from build123d import *

# Parameters (mm, degrees)
SKETCH_1_R          = 2.65
SKETCH_1_R_2        = 1.5
EXTRUDE_1_DEPTH     = 52.7
SKETCH_4_R          = 3.1
CUT_EXTRUDE_3_DEPTH = 56.399571298


with BuildPart() as part:
    # 草图1 → 凸台-拉伸1 (new, symmetric)
    with BuildSketch(Plane.XY):
        with BuildLine():
            Line((3.142893219, 3.85), (-3.142893219, 3.85))
            Line((-3.142893219, 3.85), (-5.5, 6.207106781))
            Line((-5.5, 6.207106781), (-5.5, 8.3))
            Line((-5.5, 8.3), (-3.1, 8.3))
            Line((-3.1, 8.3), (-3.1, 9.5))
            Line((-3.1, 9.5), (-3.6, 9.5))
            Line((-3.6, 9.5), (-3.6, 9.7))
            ThreePointArc((-3.6, 9.7), (-3.687867966, 9.912132034), (-3.9, 10))
            Line((-3.9, 10), (-8.5, 10))
            ThreePointArc((-8.5, 10), (-9.560660172, 9.560660172), (-10, 8.5))
            Line((-10, 8.5), (-10, 3.9))
            ThreePointArc((-10, 3.9), (-9.912132034, 3.687867966), (-9.7, 3.6))
            Line((-9.7, 3.6), (-9.5, 3.6))
            Line((-9.5, 3.6), (-9.5, 3.1))
            Line((-9.5, 3.1), (-8.3, 3.1))
            Line((-8.3, 3.1), (-8.3, 5.5))
            Line((-8.3, 5.5), (-6.207106781, 5.5))
            Line((-6.207106781, 5.5), (-3.85, 3.142893219))
            Line((-3.85, 3.142893219), (-3.85, -3.142893219))
            Line((-3.85, -3.142893219), (-6.207106781, -5.5))
            Line((-6.207106781, -5.5), (-8.3, -5.5))
            Line((-8.3, -5.5), (-8.3, -3.1))
            Line((-8.3, -3.1), (-9.5, -3.1))
            Line((-9.5, -3.1), (-9.5, -3.6))
            Line((-9.5, -3.6), (-9.7, -3.6))
            ThreePointArc((-9.7, -3.6), (-9.912132034, -3.687867966), (-10, -3.9))
            Line((-10, -3.9), (-10, -8.5))
            ThreePointArc((-10, -8.5), (-9.560660172, -9.560660172), (-8.5, -10))
            Line((-8.5, -10), (-3.9, -10))
            ThreePointArc((-3.9, -10), (-3.687867966, -9.912132034), (-3.6, -9.7))
            Line((-3.6, -9.7), (-3.6, -9.5))
            Line((-3.6, -9.5), (-3.1, -9.5))
            Line((-3.1, -9.5), (-3.1, -8.3))
            Line((-3.1, -8.3), (-5.5, -8.3))
            Line((-5.5, -8.3), (-5.5, -6.207106781))
            Line((-5.5, -6.207106781), (-3.142893219, -3.85))
            Line((-3.142893219, -3.85), (3.142893219, -3.85))
            Line((3.142893219, -3.85), (5.5, -6.207106781))
            Line((5.5, -6.207106781), (5.5, -8.3))
            Line((5.5, -8.3), (3.1, -8.3))
            Line((3.1, -8.3), (3.1, -9.5))
            Line((3.1, -9.5), (3.6, -9.5))
            Line((3.6, -9.5), (3.6, -9.7))
            ThreePointArc((3.6, -9.7), (3.687867966, -9.912132034), (3.9, -10))
            Line((3.9, -10), (8.5, -10))
            ThreePointArc((8.5, -10), (9.560660172, -9.560660172), (10, -8.5))
            Line((10, -8.5), (10, -3.9))
            ThreePointArc((10, -3.9), (9.912132034, -3.687867966), (9.7, -3.6))
            Line((9.7, -3.6), (9.5, -3.6))
            Line((9.5, -3.6), (9.5, -3.1))
            Line((9.5, -3.1), (8.3, -3.1))
            Line((8.3, -3.1), (8.3, -5.5))
            Line((8.3, -5.5), (6.207106781, -5.5))
            Line((6.207106781, -5.5), (3.85, -3.142893219))
            Line((3.85, -3.142893219), (3.85, 3.142893219))
            Line((3.85, 3.142893219), (6.207106781, 5.5))
            Line((6.207106781, 5.5), (8.3, 5.5))
            Line((8.3, 5.5), (8.3, 3.1))
            Line((8.3, 3.1), (9.5, 3.1))
            Line((9.5, 3.1), (9.5, 3.6))
            Line((9.5, 3.6), (9.7, 3.6))
            ThreePointArc((9.7, 3.6), (9.912132034, 3.687867966), (10, 3.9))
            Line((10, 3.9), (10, 8.5))
            ThreePointArc((10, 8.5), (9.560660172, 9.560660172), (8.5, 10))
            Line((8.5, 10), (3.9, 10))
            ThreePointArc((3.9, 10), (3.687867966, 9.912132034), (3.6, 9.7))
            Line((3.6, 9.7), (3.6, 9.5))
            Line((3.6, 9.5), (3.1, 9.5))
            Line((3.1, 9.5), (3.1, 8.3))
            Line((3.1, 8.3), (5.5, 8.3))
            Line((5.5, 8.3), (5.5, 6.207106781))
            Line((5.5, 6.207106781), (3.142893219, 3.85))
        make_face()
        with Locations(Location((0, 0, 0), (0, 0, 180))):
            Circle(SKETCH_1_R, mode=Mode.SUBTRACT)
        with Locations(Location((-7.75, 7.75, 0), (0, 0, 180))):
            Circle(SKETCH_1_R_2, mode=Mode.SUBTRACT)
        with Locations(Location((7.75, 7.75, 0), (0, 0, 180))):
            Circle(SKETCH_1_R_2, mode=Mode.SUBTRACT)
        with Locations(Location((7.75, -7.75, 0), (0, 0, 180))):
            Circle(SKETCH_1_R_2, mode=Mode.SUBTRACT)
        with Locations(Location((-7.75, -7.75, 0), (0, 0, 180))):
            Circle(SKETCH_1_R_2, mode=Mode.SUBTRACT)
    extrude(amount=EXTRUDE_1_DEPTH, both=True)

    # 草图4 → 切除-拉伸3 (cut, through all)
    with BuildSketch(Plane(origin=(3.85, 0, 0), x_dir=(0, 0, -1), z_dir=(1, 0, 0))):
        with Locations((-38.1, 0)):
            Circle(SKETCH_4_R)
        with Locations((38.1, 0)):
            Circle(SKETCH_4_R)
    extrude(amount=-CUT_EXTRUDE_3_DEPTH, mode=Mode.SUBTRACT)


solid = part.part
Part model, mm, in its own coordinate system. A direction names the side the tool comes from. Give positions to 0.01 mm unless a question says otherwise; leave off trailing zeros. Loops run counter-clockwise (first coordinate to the right, second up) from the corner with the lowest first, then second, coordinate; pieces in that order, holes last.
(1) Band-saw the part on B-B (x = 0). Write the cut outline in (y, z), and give its area (3 significant figures).
Return value:
outline: (-3.85, -52.7) - (-2.65, -52.7) - (-2.65, -39.71) arc R3.1 cw to (-2.65, -36.49) - (-2.65, 36.49) arc R3.1 cw to (-2.65, 39.71) - (-2.65, 52.7) - (-3.85, 52.7) - close; (2.65, -52.7) - (3.85, -52.7) - (3.85, 52.7) - (2.65, 52.7) - (2.65, 39.71) arc R3.1 cw to (2.65, 36.49) - (2.65, -36.49) arc R3.1 cw to (2.65, -39.71) - close
area: 249 mm2
(2) Pin check, flat tips, straight feed: pin 1 (8 mm diameter, centred on y = 0, z = 25, fed in from +X); pin 2 (0.6 mm diameter, centred on x = 3.5, z = 3.5, fed in from -Y). Stop position of each tip, or through.
Return value:
pin 1: stops at x = 10
pin 2: stops at y = -9.98
(3) Drill centre lines: line 1 along Y through (x, z) = (7.75, -22); line 2 along X through (y, z) = (-9, 22). Where is each one in solid material? Low to high.
Return value:
line 1: y = -10 to -9.25, -6.25 to -5.5, 5.5 to 6.25, 9.25 to 10
line 2: x = -9.91 to -8.58, -6.92 to -3.1, 3.1 to 6.92, 8.58 to 9.91
(4) Band-saw the part on C-C (z = 38.1). Count the separate pieces of the cut face and the enclosed holes in it, and give its area (3 significant figures).
Return value:
separate pieces: 2
enclosed holes: 4
area: 104 mm2
(5) Pull direction Y, two halves, no side cores. Call faces 1 (the flat face through (-10, 6, 1)), 2 (the flat face through (-5.012, -4.305, 0.738)), 3 (the flat face through (-6, 10, 1)): pulls with the +Y half, pulls with the -Y half, needs draft (parallel to the pull), parting line crosses it, or undercut.
Return value:
face 1: needs draft
face 2: undercut
face 3: pulls with the +Y half
(6) Band-saw the part on A-A (y = 0). Write the cut outline in (x, z).
Return value:
outline: (-3.85, -52.7) - (-2.65, -52.7) - (-2.65, -41.2) - (-3.85, -41.2) - close; (-3.85, -35) - (-2.65, -35) - (-2.65, 35) - (-3.85, 35) - close; (-3.85, 41.2) - (-2.65, 41.2) - (-2.65, 52.7) - (-3.85, 52.7) - close; (2.65, -52.7) - (3.85, -52.7) - (3.85, -41.2) - (2.65, -41.2) - close; (2.65, -35) - (3.85, -35) - (3.85, 35) - (2.65, 35) - close; (2.65, 41.2) - (3.85, 41.2) - (3.85, 52.7) - (2.65, 52.7) - close
(7) 3-axis set-ups, long thin cutter, end or side, ignore diameter. For faces 4 (the flat face through (10, -6, 1)), 5 (the flat face through (7, -5.5, 1)): which of +Z, -Z, +X, -X, +Y, -Y reach the whole face in a straight line?
Return value:
face 4: +Z, -Z, +X, +Y, -Y
face 5: +Z, -Z
